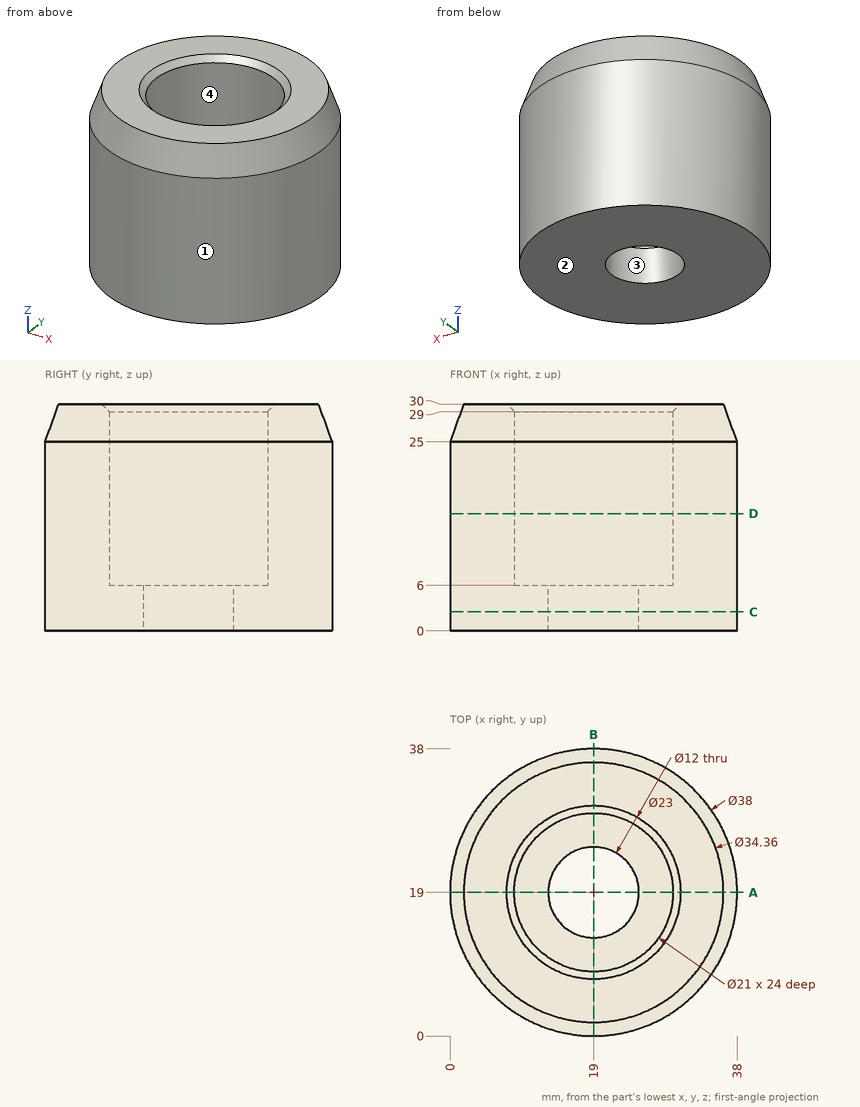
Can you work these out from the drawing? Everything is in mm from the part's minimum corner. Give positions to 0.01 mm unless a question says otherwise; leave off trailing zeros. Loops run counter-clockwise (first coordinate to the right, second up) from the corner with the lowest first, then second, coordinate; pieces in that order, holes last. Notation, with made-up numbers: M -39.5,1.5 L -16.5,1.5 A20 ccw -16.5,10.5 Z; hole C -36.75,-31.5 d9. An arc over 180 degrees is marked long. Put each result on its own line as item: value. Start each with the question number.
(1) I want a section at A-A on y = 19. Please give me the cut outline in (x, z), then the cut area to 3 significant figures.
(2) I need wall thicknesses on line 1 along Y through (x, z) = (19, 18.75); line 2 along X through (y, z) = (18.5, 18.5); line 3 along Z through (x, y) = (22.5, 11.5). Which ranges of each line are inside material? Lowest first, please. Write a range as [from, to].
(3) Will these pins go through, and if not, where does the flat tip stop? pin 1 Ø2 at (y, z) = (15.5, 15.5) entering from +X (1 decimal); pin 2 Ø15.5 at (x, y) = (19, 19) entering from +Z; pin 3 Ø6 at (y, z) = (25.5, 8) entering from +X (1 decimal).
(4) I want a section at C-C on z = 2.5. Please give me the cut outline in (x, y).
(5) I want a section at D-D on z = 15.5. Please give me the cut outline in (x, y), then the cut area to 3 significant figures.
(6) If we mould it in two halves opening along X, with no side actions, what happens to the marked faces 1, 2, 3 and 4? For each: +X half, -X half, draft (parallel to the pull), parting line (faces both ways), or undercut.
Answer block:
1. outline: M 0,0 L 13,0 L 13,6 L 8.5,6 L 8.5,29 L 7.5,30 L 1.82,30 L 0,25 Z; M 25,0 L 38,0 L 38,25 L 36.18,30 L 30.5,30 L 29.5,29 L 29.5,6 L 25,6 Z
1. area: 554 mm^2
2. line 1: [0, 8.5], [29.5, 38]
2. line 2: [0.01, 8.51], [29.49, 37.99]
2. line 3: [0, 6]
3. pin 1: x = 37.8
3. pin 2: z = 6
3. pin 3: x = 37.7
4. outline: C 19,19 d38; hole C 19,19 d12
5. outline: C 19,19 d38; hole C 19,19 d21
5. area: 788 mm^2
6. face 1: parting line
6. face 2: draft
6. face 3: undercut
6. face 4: undercut
